```python
from build123d import *

# Parameters (mm, degrees)
SKETCH1_W            = 90
SKETCH1_H            = 75
BOSS_EXTRUDE1_DEPTH  = 3
SKETCH2_W            = 90
SKETCH2_H            = 3
BOSS_EXTRUDE2_DEPTH  = 17
M5_CLEARANCE_HOLE1_D = 5.5
CUT_EXTRUDE1_REACH   = 62.994
SKETCH5_R            = 1.75


with BuildPart() as part:
    # Sketch1 → Boss-Extrude1 (new body)
    with BuildSketch(Plane(origin=(0, 0, 0), x_dir=(1, 0, 0), z_dir=(0, 1, 0))):
        Rectangle(SKETCH1_W, SKETCH1_H)
    extrude(amount=BOSS_EXTRUDE1_DEPTH)

    # Sketch2 → Boss-Extrude2 (add)
    with BuildSketch(Plane(origin=(0, 3, 0), x_dir=(1, 0, 0), z_dir=(0, 1, 0))):
        with Locations((0, 36)):
            Rectangle(SKETCH2_W, SKETCH2_H)
    extrude(amount=BOSS_EXTRUDE2_DEPTH)

    # M5 Clearance Hole1 (through all)
    with Locations(Plane(origin=(40, 10, -37.5), x_dir=(-1, 0, 0), z_dir=(0, 0, -1))):
        with Locations((0, 0), (80, 0)):
            Hole(M5_CLEARANCE_HOLE1_D / 2)

    # Sketch5 → Cut-Extrude1 (cut, up to next)
    with BuildSketch(Plane(origin=(0, 3, 0), x_dir=(1, 0, 0), z_dir=(0, 1, 0)), mode=Mode.PRIVATE) as cut_extrude1_sk1:
        with Locations(Location((-31.8, 17.55, 0), (0, 0, 270))):
            Circle(SKETCH5_R)
    cut_extrude1_tool1 = extrude(cut_extrude1_sk1.sketch, amount=-CUT_EXTRUDE1_REACH, mode=Mode.PRIVATE) & part.part
    # Sketch5 → Cut-Extrude1 (cut, up to next)
    with BuildSketch(Plane(origin=(0, 3, 0), x_dir=(1, 0, 0), z_dir=(0, 1, 0)), mode=Mode.PRIVATE) as cut_extrude1_sk2:
        with Locations(Location((-31.8, -10.35, 0), (0, 0, 270))):
            Circle(SKETCH5_R)
    cut_extrude1_tool2 = extrude(cut_extrude1_sk2.sketch, amount=-CUT_EXTRUDE1_REACH, mode=Mode.PRIVATE) & part.part
    # Sketch5 → Cut-Extrude1 (cut, up to next)
    with BuildSketch(Plane(origin=(0, 3, 0), x_dir=(1, 0, 0), z_dir=(0, 1, 0)), mode=Mode.PRIVATE) as cut_extrude1_sk3:
        with Locations(Location((19, -25.55, 0), (0, 0, 270))):
            Circle(SKETCH5_R)
    cut_extrude1_tool3 = extrude(cut_extrude1_sk3.sketch, amount=-CUT_EXTRUDE1_REACH, mode=Mode.PRIVATE) & part.part
    # Sketch5 → Cut-Extrude1 (cut, up to next)
    with BuildSketch(Plane(origin=(0, 3, 0), x_dir=(1, 0, 0), z_dir=(0, 1, 0)), mode=Mode.PRIVATE) as cut_extrude1_sk4:
        with Locations(Location((20.3, 22.65, 0), (0, 0, 270))):
            Circle(SKETCH5_R)
    cut_extrude1_tool4 = extrude(cut_extrude1_sk4.sketch, amount=-CUT_EXTRUDE1_REACH, mode=Mode.PRIVATE) & part.part
    add(cut_extrude1_tool1.solids().sort_by_distance((-31.8, 3, -17.55))[0], mode=Mode.SUBTRACT)
    add(cut_extrude1_tool2.solids().sort_by_distance((-31.8, 3, 10.35))[0], mode=Mode.SUBTRACT)
    add(cut_extrude1_tool3.solids().sort_by_distance((19, 3, 25.55))[0], mode=Mode.SUBTRACT)
    add(cut_extrude1_tool4.solids().sort_by_distance((20.3, 3, -22.65))[0], mode=Mode.SUBTRACT)


solid = part.part
```
The listing builds one solid part. Answer for the finished solid, in the listing's coordinates (mm). A direction names the side the tool comes from. Give positions to 0.01 mm unless a question says otherwise; leave off trailing zeros. Write each loop counter-clockwise with the first axis right and the second up, starting at its lowest first coordinate (ties: lowest second). Pieces come first, ordered by that corner, then holes. Notation, with made-up numbers: (23.25, 72.25) - (63.25, 72.25) arc R26 ccw to (63.25, 86.25) - close; hole circle Ø8 at (52.5, 37.5). An arc over 180 degrees is marked (long way). Use one line per item in the form item = value. Start each with the question number.
1) Find section A-A on z = -17.55. Determine the outline of the cut face in (x, y), plus the area to 4 significant figures.
2) Find section D-D on z = 25. Determine the outline of the cut face in (x, y), plus the area to 3 significant figures.
3) Flat-ended cylindrical pins translate along their axes: pin 1 Ø4 at (x, z) = (-31.8, -17.55) entering from +Y; pin 2 Ø5 at (x, y) = (-4.5, 12) entering from +Z. Find the tip coordinate at first contact, or state that the pin passes through.
4) A tool of negligible diameter and unlimited length cuts with its end or side. For faces 1 (the face through (37.253, 10.121, -35.979)), 2 (the face through (-1, 11, -34.5)), from which of +Z, -Z, +X, -X, +Y, -Y can it reach the whole face along a straight path? Write none if from no direction.
5) Find section C-C on x = -26. Determine the outline of the cut face in (y, z), plus the area to 3 significant figures.
6) The mould has two halves that part along Z. Classify faces 3 (the face through (-1, 10, -37.5)), 4 (the face through (-31.274, 1.521, 12.019)), 5 (the face through (-45, 2, -5)), 6 (the face through (20.826, 1.521, -20.981)): pulls with the +Z half, pulls with the -Z half, needs draft (parallel to the pull), parting line crosses it, or undercut.
7) Consider line 1 along Y through (x, z) = (-40, -35.2); line 2 along X through (y, z) = (0.95, 10.35); line 3 along X through (y, z) = (1.2, 25.55). Determine where each line is inside the solid, lowest interval first. Write a range as from..to.
8) Find section B-B on y = 10. Determine the outline of the cut face in (x, z), plus the area to 3 significant figures.
Geometry results:
q1.outline = (-45, 0) - (-33.55, 0) - (-33.55, 3) - (-45, 3) - close; (-30.05, 0) - (45, 0) - (45, 3) - (-30.05, 3) - close
q1.area = 259.5 mm2
q2.outline = (-45, 0) - (17.34, 0) - (17.34, 3) - (-45, 3) - close; (20.66, 0) - (45, 0) - (45, 3) - (20.66, 3) - close
q2.area = 260 mm2
q3.pin_1 = 3
q3.pin_2 = -34.5
q4.face_1 = +Z, -Z
q4.face_2 = +Z, +X, -X, +Y
q5.outline = (0, -37.5) - (20, -37.5) - (20, -34.5) - (3, -34.5) - (3, 37.5) - (0, 37.5) - close
q5.area = 276 mm2
q6.face_3 = pulls with the -Z half
q6.face_4 = undercut
q6.face_5 = needs draft
q6.face_6 = undercut
q7.line_1 = 0..7.25, 12.75..20
q7.line_2 = -45..-33.55, -30.05..45
q7.line_3 = -45..17.25, 20.75..45
q8.outline = (-45, -37.5) - (-42.75, -37.5) - (-42.75, -34.5) - (-45, -34.5) - close; (-37.25, -37.5) - (37.25, -37.5) - (37.25, -34.5) - (-37.25, -34.5) - close; (42.75, -37.5) - (45, -37.5) - (45, -34.5) - (42.75, -34.5) - close
q8.area = 237 mm2
